Geometry check sheet. Reference: the model listing, model coordinates, mm. Face numbers are marked on the shaded views. A direction names the side the tool comes from. Round coordinates to 2 decimals unless told otherwise and drop trailing zeros. Order: outer loops, then holes, each group sorted by start corner. A loop starts at its lowest first (then second) coordinate and runs counter-clockwise, first axis right, second up.
(1) Thickness scan on L1, parallel to X at y = 13.25, z = 30; L2, parallel to X at y = 13.5, z = 63; L3, parallel to Y at x = 25, z = 44. Record the ranges inside material, lowest first.
(2) Gauge pin test, flat ends, axial feed: P1, Ø10, axis at y = 7, z = 47.5, coming from the -X side; P2, Ø3, axis at x = 37, z = 85, coming from the -Y side; P3, Ø5, axis at y = 12.5, z = 32.5, coming from the +X side. Record the tip position at first contact, or that the pin passes through.
(3) Set-up check for the marked faces 1 and 2: record each of +Z, -Z, +X, -X, +Y, -Y from which the full face is reachable in a straight line by a thin tool's end or side.
(4) Cross-section at A-A on z = 86.5. Enter the section's corners in (x, y), and give its area (3 significant figures).
(5) Cross-section at C-C on x = 14. Count the separate pieces of the cut face and the enclosed holes in it, and give its area (3 significant figures).
(6) Cross-section at B-B on y = 15.25. Enter the section's corners in (x, z), and give its area (3 significant figures).
from build123d import *

# Parameters (mm, degrees)
BOSS_EXTRUDE1_DEPTH     = 101.6
SKETCH4_R               = 3.9751
CUT_EXTRUDE3_DEPTH      = 114.32570869
ESQUISSE1_R             = 3.9751
ENL_V_MAT_EXTRU_1_DEPTH = 107.941428186


with BuildPart() as part:
    # Sketch1 → Boss-Extrude1 (new body)
    with BuildSketch(Plane.XY):
        Polygon((0, 0), (22.450640303, 22.450640303), (44.901280605, 0), (42.656216575, -2.24506403), (22.450640303, 17.960512242), (2.24506403, -2.24506403), align=None)
    extrude(amount=BOSS_EXTRUDE1_DEPTH)

    # Sketch4 → Cut-Extrude3 (cut, through all)
    with BuildSketch(Plane(origin=(0, 0, 0), x_dir=(0, 0, 1), z_dir=(-0.7071067811865476, 0.7071067811865475, 0))):
        with Locations(Location((31.75, 15.875, 0), (0, 0, 270))):
            Circle(SKETCH4_R)
        with Locations(Location((69.85, 15.875, 0), (0, 0, 270))):
            Circle(SKETCH4_R)
    extrude(amount=-CUT_EXTRUDE3_DEPTH, mode=Mode.SUBTRACT)

    # Esquisse1 → Enlèv. mat.-Extru.1 (cut, through all)
    with BuildSketch(Plane(origin=(22.450640303, 22.450640303, 0), x_dir=(-0.7071067811865476, 0.7071067811865475, 0), z_dir=(0.7071067811865475, 0.7071067811865476, 0))):
        with Locations((-15.875, 12.7)):
            Circle(ESQUISSE1_R)
    enl_v_mat_extru_1 = extrude(amount=-ENL_V_MAT_EXTRU_1_DEPTH, mode=Mode.SUBTRACT)

    # Symétrie1: Enlèv. mat.-Extru.1 across plane
    add(enl_v_mat_extru_1.mirror(Plane.XY.offset(50.8)), mode=Mode.SUBTRACT)


solid = part.part
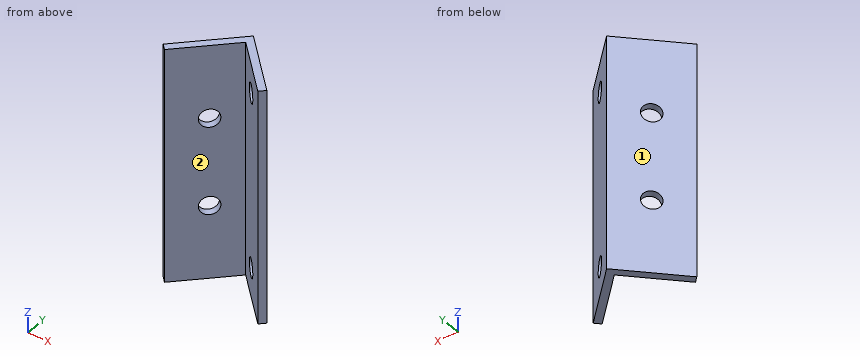
Found:
1. L1: x = 14.25 to 17.74, 27.16 to 31.65
1. L2: x = 13.5 to 17.99, 26.91 to 31.4
1. L3: y = 15.41 to 19.9
2. P1: stops at x = 2
2. P2: stops at y = 1.91
2. P3: stops at x = 34.9
3. face 1: +Z, -Z, -X, +Y
3. face 2: +Z, -Z, -Y
4. outline: (0, 0) - (2.25, -2.25) - (22.45, 17.96) - (29.19, 11.22) - (31.44, 13.47) - (22.45, 22.45) - close; (33.67, 6.74) - (42.66, -2.25) - (44.9, 0) - (35.92, 8.98) - close
4. area: 171 mm2
5. separate pieces: 3
5. enclosed holes: 0
5. area: 403 mm2
6. outline: (15.25, 0) - (19.74, 0) - (19.74, 101.6) - (15.25, 101.6) - close; (25.16, 0) - (29.65, 0) - (29.65, 101.6) - (25.16, 101.6) - close
6. area: 912 mm2
